Verification items for this drawing (mm, ordinates from the low corner). A direction names the side the tool comes from. Give positions to 0.01 mm unless a question says otherwise; leave off trailing zeros. Write each loop counter-clockwise with the first axis right and the second up, starting at its lowest first coordinate (ties: lowest second). Pieces come first, ordered by that corner, then holes. Notation, with made-up numbers: (-2.75, -2) -> (36.25, -2) arc R15 cw to (36.25, 15) -> close; hole circle Ø3 at (-18.75, 79.5). An arc over 180 degrees is marked (long way). One line per item, written item: value.
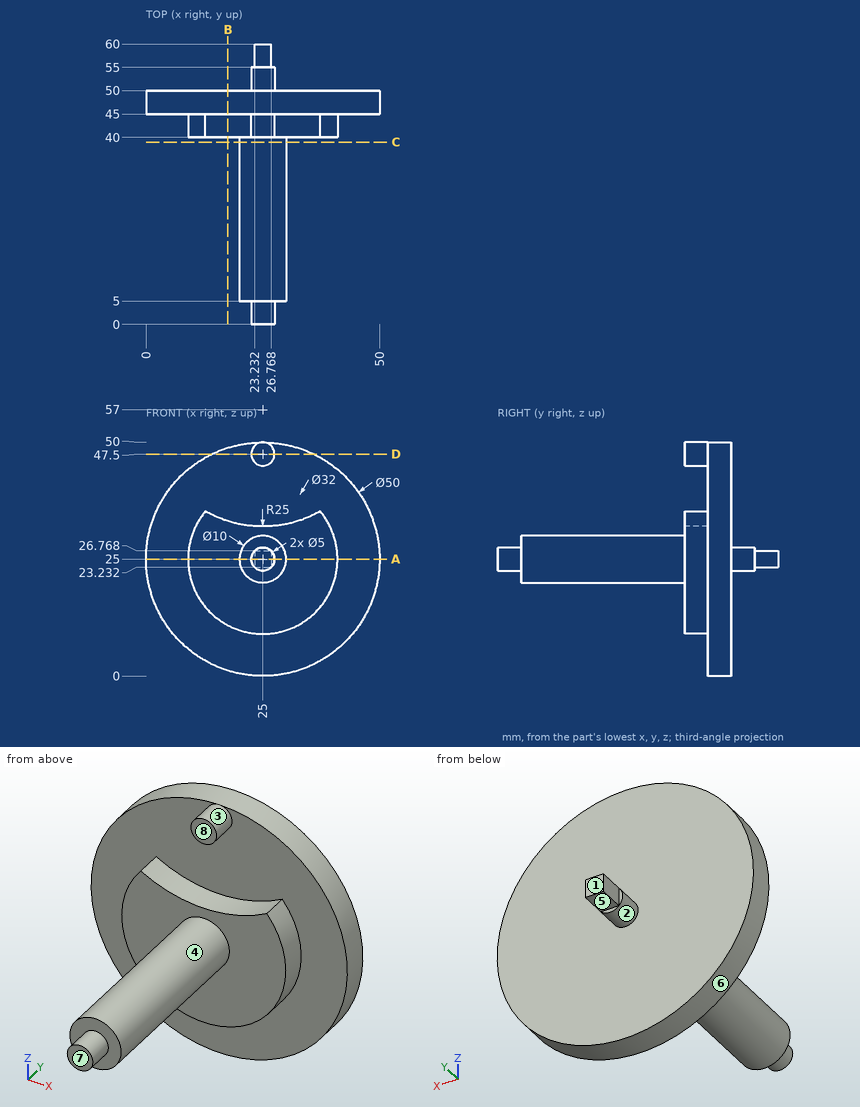
1) Sectioned sample at D-D on z = 47.5. Record the cut outline in (x, y), plus the area to 3 significant figures.
Verdict:
outline: (14.1, 45) -> (22.5, 45) -> (22.5, 40) -> (27.5, 40) -> (27.5, 45) -> (35.9, 45) -> (35.9, 50) -> (14.1, 50) -> close
area: 134 mm^2
2) Sectioned sample at A-A on z = 25. Record the cut outline in (x, y).
Verdict:
outline: (0, 45) -> (9, 45) -> (9, 40) -> (20, 40) -> (20, 5) -> (22.5, 5) -> (22.5, 0) -> (27.5, 0) -> (27.5, 5) -> (30, 5) -> (30, 40) -> (41, 40) -> (41, 45) -> (50, 45) -> (50, 50) -> (27.5, 50) -> (27.5, 55) -> (26.77, 55) -> (26.77, 60) -> (23.23, 60) -> (23.23, 55) -> (22.5, 55) -> (22.5, 50) -> (0, 50) -> close
3) Sectioned sample at C-C on y = 39. Record the cut outline in (x, z).
Verdict:
outline: circle Ø10 at (25, 25)
4) Depth check by flat-ended pin: pin 1 Ø1.8 at (x, y) = (24.5, 56.5) entering from +Z; pin 2 Ø6 at (x, z) = (32, 16.5) entering from -Y; pin 3 Ø8 at (x, y) = (38.5, 46) entering from +Z (1 decimal). Enter the tip coordinate at first touch or a pass-through.
Verdict:
pin 1: z = 26.77
pin 2: y = 40
pin 3: z = 48.1
5) Mould release check, pull along Z, two halves, no side actions. Record for the marked faces 1, 2 and 3: released by +Z, released by -Z, zero draft, split by the parting line, or undercut.
Verdict:
face 1: zero draft
face 2: split by the parting line
face 3: undercut
6) Sectioned sample at B-B on x = 17.5. Record the cut outline in (y, z), plus the area to 3 significant figures.
Verdict:
outline: (40, 10.87) -> (45, 10.87) -> (45, 1.15) -> (50, 1.15) -> (50, 48.85) -> (45, 48.85) -> (45, 33.15) -> (40, 33.15) -> close
area: 350 mm^2
7) Scan lines: probe 1 along Y at (x, z) = (42, 37); probe 2 along Y at (x, z) = (11, 21.5); probe 3 along Z at (x, y) = (21.5, 6.5). Record each from-to range of solid material in increasing order.
Verdict:
probe 1: 45 to 50
probe 2: 40 to 50
probe 3: 21.43 to 28.57
8) Tool access check on the marked faces 4, 5, 6, 7 and 8. Record the directions out of +Z, -Z, +X, -X, +Y, -Y that give a thin tool (end or side, any length) a straight path to the whole face; none if there is none.
Verdict:
face 4: -Y
face 5: -Z, +X, -X, +Y
face 6: +Y, -Y
face 7: +Z, -Z, +X, -X, -Y
face 8: +Z, +X, -X, -Y
